Build history of the part. All positions in model axes, mm. Face numbers are marked on the shaded views. A direction names the side the tool comes from. Coordinates: 2 decimals unless noted, no trailing zeros. Loops run counter-clockwise (first coordinate to the right, second up) from the corner with the lowest first, then second, coordinate; pieces in that order, holes last.
Item 1: 3-axis set-ups, long thin cutter, end or side, ignore diameter. For the marked faces 1 and 2: which of +Z, -Z, +X, -X, +Y, -Y reach the whole face in a straight line?
Item 2: Cut at C-C (z = -1). List the corners of the cut face in (x, y), and give its area (3 significant figures).
Item 3: Cut at A-A (z = 1.5). List the corners of the cut face in (x, y).
Item 4: Cut at B-B (z = 3.25). List the corners of the cut face in (x, y), and give its area (3 significant figures).
Item 5: Flat gauge pins, fed straight in: pin 1 (0.9 mm diameter, centred on x = -2, y = 2, fed in from -Z); pin 2 (1.1 mm diameter, centred on x = 0, y = 3.5, fed in from -Z); pin 3 (1.4 mm diameter, centred on x = 3, y = 1, fed in from -Z). Where does each tip first touch, or does it go through?
Item 6: Drill centre lines: line 1 along Y through (x, z) = (0, 5.05); line 2 along X through (y, z) = (-0.25, 2.75); line 3 along X through (y, z) = (0, -1.8). Where is each one in solid material? Low to high.
from build123d import *

# Parameters (mm, degrees)
F2_DEPTH  = 3
F3_R      = 2.3865
F4_DEPTH  = 5
F8_D      = 3
F8_DEPTH  = 6
F10_D     = 0.4
F10_DEPTH = 6


with BuildPart() as f2:
    # F1 (on Top) → F2 (new body)
    with BuildSketch(Plane.XY):
        Polygon((3.5, -2.020726), (3.5, 2.020726), (0, 4.041452), (-3.5, 2.020726), (-3.5, -2.020726), (0, -4.041452), align=None)
    extrude(amount=F2_DEPTH)

    # F3 (on face) → F4 (join)
    with BuildSketch(Plane.XY.offset(3)):
        Circle(F3_R)
    extrude(amount=F4_DEPTH)

    # F5 (on Front) → F6 (revolve)
    with BuildSketch(Plane.XZ):
        Polygon((0, -2), (0, 0), (-3.5, 0), (-0.6, -2), align=None)
    revolve(axis=Axis((0, 0, -1), (0, 0, 1)))

    # F8
    with Locations(Plane.XY.offset(8)):
        with Locations((0, 0)):
            Hole(F8_D / 2, depth=F8_DEPTH)

    # F10
    with Locations(Plane(origin=(0, 0, -2), x_dir=(1, 0, 0), z_dir=(0, 0, -1))):
        with Locations((0, 0)):
            Hole(F10_D / 2, depth=F10_DEPTH)

    # F11 (on Front) → F12 (revolve, cut)
    with BuildSketch(Plane.XZ):
        Polygon((0, 2), (-1.5, 2), (-0.2, -1.4), (0, -1.4), align=None)
    revolve(axis=Axis((0, 0, 0.3), (0, 0, -1)), mode=Mode.SUBTRACT)


solid = f2.part
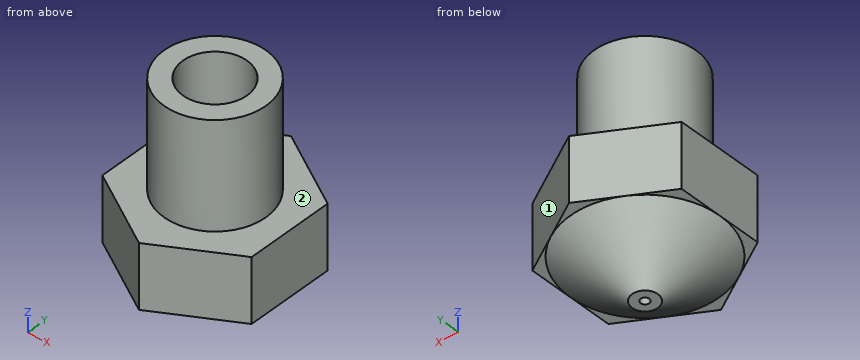
Filled sheet:
1. face 1: +Z, -Z, +X, +Y
1. face 2: +Z
2. outline: circle Ø4.1 at (0, 0); hole circle Ø0.71 at (0, 0)
2. area: 12.8 mm2
3. outline: (-3.5, -2.02) - (0, -4.04) - (3.5, -2.02) - (3.5, 2.02) - (0, 4.04) - (-3.5, 2.02) - close; hole circle Ø2.62 at (0, 0)
4. outline: circle Ø4.77 at (0, 0); hole circle Ø3 at (0, 0)
4. area: 10.8 mm2
5. pin 1: stops at z = -0.77
5. pin 2: stops at z = -0.38
5. pin 3: stops at z = -0.72
6. line 1: y = -2.39 to -1.5, 1.5 to 2.39
6. line 2: x = -3.5 to -1.48, 1.48 to 3.5
6. line 3: x = -0.89 to -0.2, 0.2 to 0.89
